Autodesk Inventor part; units mm, degrees
ref_plane "YZ Plane" through (0, 0, 0) normal (1, 0, 0) x (0, 1, 0)
ref_plane "XZ Plane" through (0, 0, 0) normal (0, 1, 0) x (-1, 0, 0)
ref_plane "XY Plane" through (0, 0, 0) normal (0, 0, 1) x (1, 0, 0)
sketch "Sketch1" plane through (0, 0, 0) normal (0, 1, 0) x (-1, 0, 0)
  circle A0 centre (0, 0) radius 2.1
  circle A1 centre (0, 46) radius 2.1
  circle A2 centre (0, -39) radius 2.6
  circle A3 centre (66, -39) radius 2.6
  circle A4 centre (46, -22.7383) radius 2.6
  circle A5 centre (66, -22.7383) radius 2.6
  circle A6 centre (44, -39) radius 2.6
  circle A7 centre (22, -39) radius 2.6
  line L0 (0, 23) -> (66, 23) construction
  circle A8 centre (0, 85) radius 2.6
  circle A9 centre (66, 85) radius 2.6
  circle A10 centre (46, 68.7383) radius 2.6
  circle A11 centre (66, 68.7383) radius 2.6
  circle A12 centre (44, 85) radius 2.6
  circle A13 centre (22, 85) radius 2.6
  circle A14 centre (66, -39) radius 7.3625 construction
  circle A15 centre (66, 85) radius 7.3625 construction
  circle A16 centre (0, 85) radius 7.3625 construction
  circle A17 centre (0, -39) radius 7.3625 construction
  line L1 (73.3625, -39) -> (73.3625, 85)
  line L2 (66, -46.3625) -> (0, -46.3625)
  line L3 (-7.3625, -39) -> (-7.3625, 85)
  line L4 (0, 92.3625) -> (66, 92.3625)
  arc A18 (66, -46.3625) -> (73.3625, -39) centre (66, -39) ccw
  arc A19 (-7.3625, -39) -> (0, -46.3625) centre (0, -39) ccw
  arc A20 (0, 92.3625) -> (-7.3625, 85) centre (0, 85) ccw
  arc A21 (73.3625, 85) -> (66, 92.3625) centre (66, 85) ccw
  dimension "d0" = 4.2
  dimension "d1" = 46
  dimension "d2" = 39
  dimension "d3" = 66
  dimension "d4" = 20
  dimension "d6" = 22
  dimension "d7" = 22
  dimension "d8" = 23
  dimension "d9" = 4.7625
  dimension "d12" = 91.4766
  dimension "d13" = 5.2
extrude "Extrusion1" add sketch "Sketch1" along normal blind 4.7625
equation "\"d6\" = 0.333333 * d3"
equation "\"d7\" = d6"
equation "\"d8\" = 0.5 * d1"
properties part number "CNC-016-SpindleMountPlate" material "Aluminum 6061"
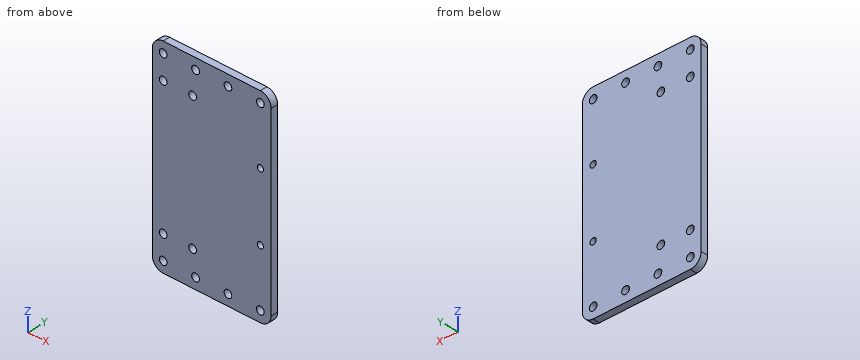
The listing builds one solid part. Answer for the finished solid, in the listing's coordinates (mm). Coordinates: 2 decimals unless noted, no trailing zeros. Loops run counter-clockwise (first coordinate to the right, second up) from the corner with the lowest first, then second, coordinate; pieces in that order, holes last. Notation, with made-up numbers: (65, 59.5) -> (82, 59.5) arc R36 ccw to (82, 96.5) -> close; hole circle Ø8 at (-21, 41). An arc over 180 degrees is marked (long way). Answer in a Markdown table with one row per item. Add a question column.
1. Consider line 1 (Z direction, x = -66, y = 1.6); line 2 (Z direction, x = 0, y = 3); line 3 (X direction, y = 4.3, z = -23). Determine where each line is inside the solid, lowest interval first. Write a range as [from, to].
2. A flat-ended cylindrical pin translates along its axis: P1, Ø4.5, axis at x = -46, z = -22.74, coming from the -Y side. Find the tip coordinate at first contact, or state that the pin passes through.
3. The part is cut by section C-C, the plane y = 1.5. Count the separate pieces of the cut face and the enclosed holes in it, then the cut area to 3 significant figures.
4. The part is cut by section B-B, the plane x = -22. Write down the section's boundary in (y, z), then the cut area to 3 significant figures.
5. The part is cut by section A-A, the plane z = 0. Write down the section's boundary in (x, y), then the cut area to 3 significant figures.
Answer below:
| question | item | result |
|---|---|---|
| 1 | line 1 | [-46.36, -41.6], [-36.4, -25.34], [-20.14, 66.14], [71.34, 82.4], [87.6, 92.36] |
| 1 | line 2 | [-46.36, -41.6], [-36.4, -2.1], [2.1, 43.9], [48.1, 82.4], [87.6, 92.36] |
| 1 | line 3 | [-73.36, -68.59], [-63.41, -48.59], [-43.41, 7.36] |
| 2 | P1 | through |
| 3 | separate pieces | 1 |
| 3 | enclosed holes | 14 |
| 3 | area | 10,900 mm2 |
| 4 | outline | (0, -46.36) -> (4.76, -46.36) -> (4.76, -41.6) -> (0, -41.6) -> close; (0, -36.4) -> (4.76, -36.4) -> (4.76, 82.4) -> (0, 82.4) -> close; (0, 87.6) -> (4.76, 87.6) -> (4.76, 92.36) -> (0, 92.36) -> close |
| 4 | area | 611 mm2 |
| 5 | outline | (-73.36, 0) -> (-2.1, 0) -> (-2.1, 4.76) -> (-73.36, 4.76) -> close; (2.1, 0) -> (7.36, 0) -> (7.36, 4.76) -> (2.1, 4.76) -> close |
| 5 | area | 364 mm2 |
